```python
from build123d import *

# Parameters (mm, degrees)
SKETCH1_W           = 8
SKETCH1_H           = 10
SKETCH1_R           = 2
BOSS_EXTRUDE1_DEPTH = 20.5
SKETCH1_3_R         = 2
CUT_EXTRUDE1_DEPTH  = 23
SKETCH2_R           = 1.625
CUT_EXTRUDE3_DEPTH  = 12
CHAMFER1_SIZE       = 0.5
SKETCH3_R           = 3
CUT_EXTRUDE4_DEPTH  = 1.5


with BuildPart() as part:
    # Sketch1 → Boss-Extrude1 (new body)
    # profile 1 of 2: a face of its own
    with BuildSketch(Plane.XY):
        Rectangle(SKETCH1_W, SKETCH1_H)
        Circle(SKETCH1_R, mode=Mode.SUBTRACT)
    # profile 2 of 2: a face of its own
    with BuildSketch(Plane.XY):
        Circle(SKETCH1_R)
    extrude(amount=BOSS_EXTRUDE1_DEPTH)

    # Sketch1_3 → Cut-Extrude1 (cut)
    with BuildSketch(Plane.XY):
        Circle(SKETCH1_3_R)
    extrude(amount=CUT_EXTRUDE1_DEPTH, mode=Mode.SUBTRACT)

    # Sketch2 → Cut-Extrude3 (cut)
    with BuildSketch(Plane(origin=(0, 5, 0), x_dir=(1, 0, 0), z_dir=(0, 1, 0))):
        with Locations(Location((0, -10.25, 0), (0, 0, 270))):
            Circle(SKETCH2_R)
    extrude(amount=-CUT_EXTRUDE3_DEPTH, mode=Mode.SUBTRACT)

    # Chamfer1
    chamfer1_edges = [part.edges().sort_by_distance(p)[0] for p in [
        (0, 5, 20.5),
        (-4, 0, 20.5),
        (0, -5, 20.5),
        (4, 0, 20.5),
        (0, -5, 0),
        (-4, 0, 0),
        (0, 5, 0),
        (4, 0, 0),
        (4, -5, 10.25),
        (-4, -5, 10.25),
        (-4, 5, 10.25),
        (4, 5, 10.25),
    ]]
    chamfer(chamfer1_edges, length=CHAMFER1_SIZE)

    # Sketch3 → Cut-Extrude4 (cut)
    with BuildSketch(Plane(origin=(0, 5, 0), x_dir=(1, 0, 0), z_dir=(0, 1, 0))):
        with Locations(Location((0, -10.25, 0), (0, 0, 270))):
            Circle(SKETCH3_R)
    extrude(amount=-CUT_EXTRUDE4_DEPTH, mode=Mode.SUBTRACT)


solid = part.part
```
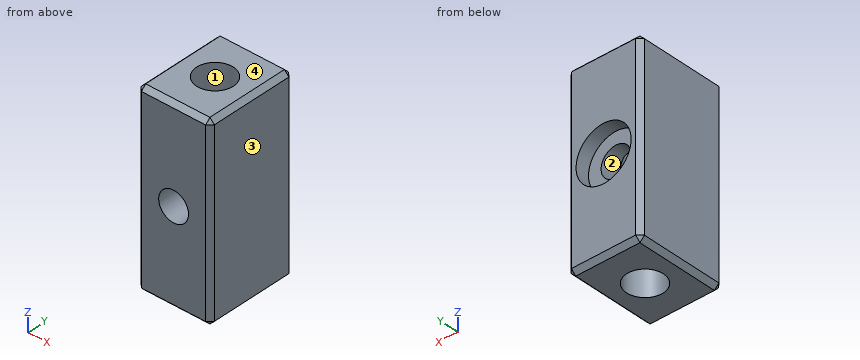
Verification items for the finished model (mm, model axes). Face numbers are marked on the shaded views. Give positions to 0.01 mm unless a question says otherwise; leave off trailing zeros. Order: outer loops, then holes, each group sorted by start corner. A loop starts at its lowest first (then second) coordinate and runs counter-clockwise, first axis right, second up. Notation, with made-up numbers: M 79.25,6.25 L 98.25,6.25 A16 cw 98.25,28.25 Z; hole C 17.5,-5.75 d3. An arc over 180 degrees is marked long. Return JSON: item names as keys, results as strings. Group by question number.
1) Section check D-D on z = 10.25. Record the cut outline in (x, y) (3 decimals).
2) Mould release check, pull along X, two halves, no side actions. Record for the marked faces 1, 2, 3 and 4: pulls with the +X half, pulls with the -X half, needs draft (parallel to the pull), parting line crosses it, or undercut.
3) Section check B-B on x = 0. Record the cut outline in (y, z) (3 decimals).
4) Section check C-C on z = 18. Record the cut outline in (x, y), and give its area (3 significant figures).
5) Section check A-A on y = 0. Record the cut outline in (x, z).
6) Go/stop test with a flat-tipped pin: pin 1 Ø1.8 at (x, z) = (0.5, 11.5) entering from +Y. Record where the tip stops, or that it passes through.
7) Scan lines: line 1 (Z direction, x = 0, y = 2.15) (3 decimals); line 2 (X direction, y = 2.05, z = 10.25) (3 decimals); line 3 (X direction, y = 0, z = 13). Record each from-to range of solid material in increasing order.
Answer block:
{
 "1": {"outline": "M -4,-4.5 L -3.5,-5 L -1.625,-5 L -1.625,-1.166 A2 cw -1.625,1.166 L -1.625,3.5 L -3,3.5 L -3,5 L -3.5,5 L -4,4.5 Z; M 1.625,-5 L 3.5,-5 L 4,-4.5 L 4,4.5 L 3.5,5 L 3,5 L 3,3.5 L 1.625,3.5 L 1.625,1.166 A2 cw 1.625,-1.166 Z"},
 "2": {"face 1": "undercut", "face 2": "undercut", "face 3": "pulls with the +X half", "face 4": "needs draft"},
 "3": {"outline": "M -5,0.5 L -4.5,0 L -2,0 L -2,8.625 L -5,8.625 Z; M -5,11.875 L -2,11.875 L -2,20.5 L -4.5,20.5 L -5,20 Z; M 2,0 L 4.5,0 L 5,0.5 L 5,7.25 L 3.5,7.25 L 3.5,8.625 L 2,8.625 Z; M 2,11.875 L 3.5,11.875 L 3.5,13.25 L 5,13.25 L 5,20 L 4.5,20.5 L 2,20.5 Z"},
 "4": {"outline": "M -4,-4.5 L -3.5,-5 L 3.5,-5 L 4,-4.5 L 4,4.5 L 3.5,5 L -3.5,5 L -4,4.5 Z; hole C 0,0 d4", "area": "66.9 mm^2"},
 "5": {"outline": "M -4,0.5 L -3.5,0 L -2,0 L -2,20.5 L -3.5,20.5 L -4,20 Z; M 2,0 L 3.5,0 L 4,0.5 L 4,20 L 3.5,20.5 L 2,20.5 Z"},
 "6": {"pin 1": "stops at y = 3.5"},
 "7": {"line 1": "z = 0 to 8.625, 11.875 to 20.5", "line 2": "x = -4 to -1.625, 1.625 to 4", "line 3": "x = -4 to -2, 2 to 4"}
}
